The drawing under review shows one solid part. Ordinate dimensions are in mm from its lowest x, y, z. A direction names the side the tool comes from. Round coordinates to 2 decimals unless told otherwise and drop trailing zeros. Loops run counter-clockwise (first coordinate to the right, second up) from the corner with the lowest first, then second, coordinate; pieces in that order, holes last. Notation, with made-up numbers: M -19,57 L 20,57 A26 cw 20,84 Z; hole C -36,41.5 d10. An arc over 180 degrees is marked long. Use a Markdown table: item, result.
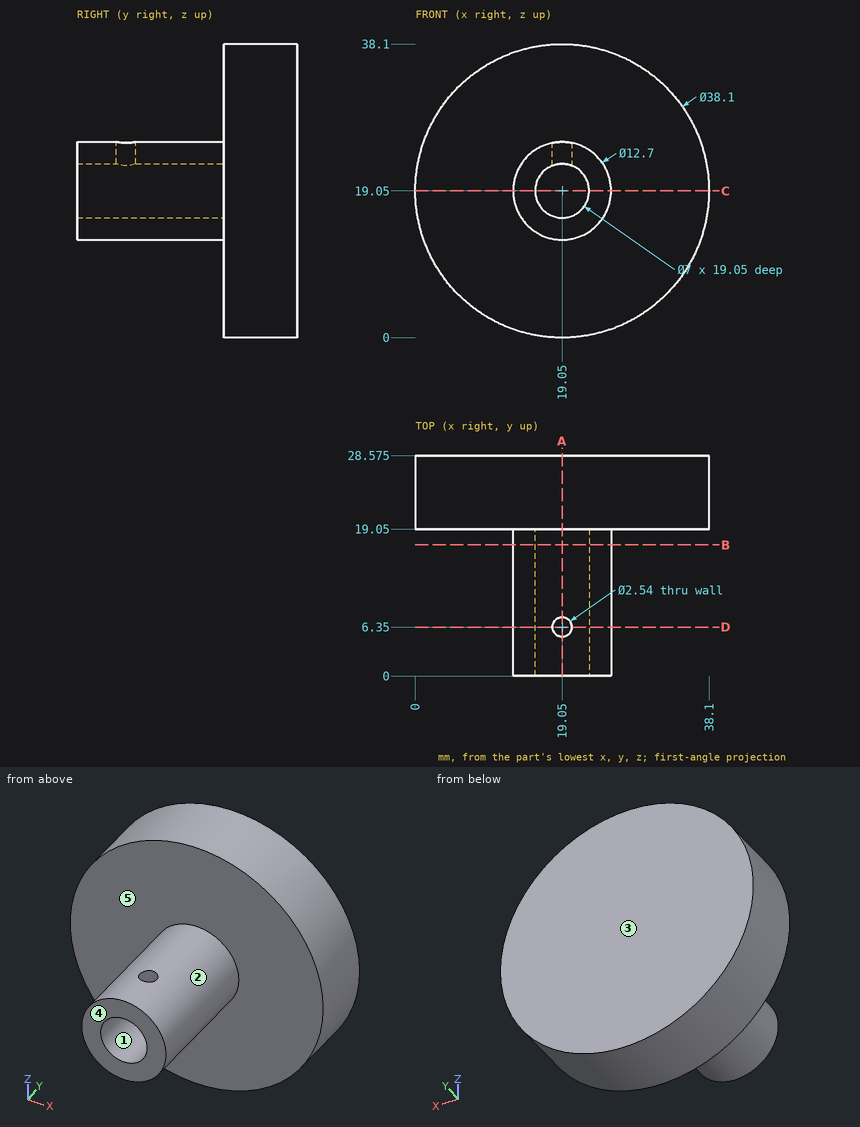
1. Take a section at A-A on x = 19.05. Give the boundary of the cut face in (y, z) (3 decimals).
Check values:
| item | result |
|---|---|
| outline | M 0,12.7 L 19.05,12.7 L 19.05,0 L 28.575,0 L 28.575,38.1 L 19.05,38.1 L 19.05,25.4 L 7.62,25.4 L 7.62,22.55 L 19.05,22.55 L 19.05,15.55 L 0,15.55 Z; M 0,22.55 L 5.08,22.55 L 5.08,25.4 L 0,25.4 Z |
2. Insertion check: pin 1 (3 mm diameter, centred on y = 18.5, z = 26, fed in from -X); pin 2 (9 mm diameter, centred on x = 19.05, z = 19.05, fed in from -Y); pin 3 (6 mm diameter, centred on x = 13.5, y = 21.5, fed in from -Z); pin 4 (6 mm diameter, centred on x = 34, z = 14.5, fed in from -Y). Each pin has a flat end and moves straight along its axis. Give the tip position at first contact, or say it passes through.
Check values:
| item | result |
|---|---|
| pin 1 | stops at x = 0.83 |
| pin 2 | stops at y = 0 |
| pin 3 | stops at z = 0.17 |
| pin 4 | stops at y = 19.05 |
3. Take a section at C-C on z = 19.05. Give the boundary of the cut face in (x, y) (3 decimals).
Check values:
| item | result |
|---|---|
| outline | M 0,19.05 L 12.7,19.05 L 12.7,0 L 15.55,0 L 15.55,19.05 L 22.55,19.05 L 22.55,0 L 25.4,0 L 25.4,19.05 L 38.1,19.05 L 38.1,28.575 L 0,28.575 Z |
4. Take a section at B-B on y = 17. Give the boundary of the cut face in (x, z).
Check values:
| item | result |
|---|---|
| outline | C 19.05,19.05 d12.7; hole C 19.05,19.05 d7 |
5. Machinability: for the marked faces 4 and 5, which of the approach directions +Z, -Z, +X, -X, +Y, -Y give a long, thin tool a straight path to every point of the face, cutting with its end or side? Answer none if there is none.
Check values:
| item | result |
|---|---|
| face 4 | +Z, -Z, +X, -X, -Y |
| face 5 | -Y |
6. Take a section at D-D on y = 6.35. Give the boundary of the cut face in (x, z), and give its area (3 significant figures).
Check values:
| item | result |
|---|---|
| outline | M 17.78,22.31 L 17.78,25.27 A6.35 ccw long 20.32,25.27 L 20.32,22.31 A3.5 cw long Z |
| area | 80.9 mm² |
7. The part is to be moulded in two halves that separate along Z. For the marked faces 1, 2 and 3, say which applies: pulls with the +Z half, pulls with the -Z half, needs draft (parallel to the pull), parting line crosses it, or undercut.
Check values:
| item | result |
|---|---|
| face 1 | undercut |
| face 2 | parting line crosses it |
| face 3 | needs draft |
8. Wall thickness on line 1 along Z through (x, y) = (19.05, 13.5); line 2 along Y through (x, z) = (19.05, 23.45) (3 decimals); line 3 along Y through (x, z) = (14.5, 8) (3 decimals): over which ranges is each line inside the solid? List them lowest first. Write a range as from..to.
Check values:
| item | result |
|---|---|
| line 1 | z = 12.7..15.55, 22.55..25.4 |
| line 2 | y = 0..5.08, 7.62..28.575 |
| line 3 | y = 19.05..28.575 |
